Input: part model. Units: mm. Frame: model coordinates. A direction names the side the tool comes from. Give positions to 0.01 mm unless a question says otherwise; leave off trailing zeros. Loops run counter-clockwise (first coordinate to the right, second up) from the corner with the lowest first, then second, coordinate; pieces in that order, holes last. Notation, with made-up numbers: M 44.25,87 L 48.25,87 A23 cw 48.25,110 Z; hole C 58.5,25 d7. An arc over 180 degrees is marked long. One line per item, written item: value. Start each with the question number.
(1) Pin query (flat end, axial travel): P1, Ø0.9, axis at y = 2.5, z = 2, coming from the -X side; P2, Ø1.5, axis at x = 1.5, z = -1, coming from the +Y side; P3, Ø1.2, axis at x = -2.54, y = -4.43, coming from the -Z side. Return the tip coordinate at first contact, or that it passes through.
(2) Section C-C on x = -1. Output: boundary loops of the cut face in (y, z).
(3) Section B-B on y = -4.43. Output: boundary loops of the cut face in (x, z).
(4) Ray query, line 1 along Y through (x, z) = (0, 0.6); line 2 along X through (y, z) = (3.75, -1.05); line 3 along Z through (x, y) = (-2.25, -3). Return the intervals inside material, ascending. Write a range as from..to.
(5) Access query for faces 4 (the flat face through (0, 5.2, -1)), 5 (the flat face through (-3.3, 2, 2)), 6 (the flat face through (3.3, 2, -1)). Directions: +Z, -Z, +X, -X, +Y, -Y. A direction counts if a zero-diameter tool reaches every point of the face in a straight line with its end or side. Return the directions, or none.
(6) Section A-A on x = 0. Output: boundary loops of the cut face in (y, z), plus the area to 3 significant figures.
(7) Pull-direction query (X, two-part tool) for faces 1 (the flat face through (-3.3, 2, -1)), 2 (the cylindrical face through (-2.65, -3.93, 0.5)), 3 (the flat face through (0, 2, 2.82)); classes: released by +X, released by -X, zero draft, split by the parting line, or undercut.
(8) Section D-D on z = 2.4. Output: boundary loops of the cut face in (x, y).
Autodesk Inventor part; units mm, degrees
ref_plane "YZ Plane" through (0, 0, 0) normal (1, 0, 0) x (0, 1, 0)
ref_plane "XZ Plane" through (0, 0, 0) normal (0, 1, 0) x (-1, 0, 0)
ref_plane "XY Plane" through (0, 0, 0) normal (0, 0, 1) x (1, 0, 0)
sketch "スケッチ1" plane through (0, 0, 0) normal (0, 0, 1) x (1, 0, 0)
  line L0 (-3.8, -5.7) -> (3.8, -5.7)
  line L1 (3.8, -5.7) -> (3.8, 5.7)
  line L2 (3.8, 5.7) -> (-3.8, 5.7)
  line L3 (-3.8, 5.7) -> (-3.8, -5.7)
  line L4 (-3.8, -5.7) -> (3.8, 5.7) construction
  line L5 (3.8, -5.7) -> (-3.8, 5.7) construction
  circle A0 centre (0, -4.43) radius 0.51
  circle A1 centre (-2.54, -4.43) radius 0.51
  circle A2 centre (2.54, -4.43) radius 0.51
  point P0 (0, 0)
  point P1 (0, 0)
  dimension "d0" = 11.4
  dimension "d1" = 7.6
  dimension "d2" = 1.27
  dimension "d3" = 2.54
  dimension "d4" = 2.54
  dimension "d5" = 1.02
extrude "押し出し1" add sketch "スケッチ1" along normal blind 1.02
sketch "スケッチ2" plane through (0, 0, 1.02) normal (0, 0, 1) x (1, 0, 0)
  line L0 (-3.3, 5.2) -> (3.3, 5.2)
  line L1 (3.3, 5.2) -> (3.3, -0.8)
  line L2 (3.3, -0.8) -> (-3.3, -0.8)
  line L3 (-3.3, -0.8) -> (-3.3, 5.2)
  line L4 (-3.3, 5.2) -> (3.3, -0.8) construction
  line L5 (3.3, 5.2) -> (-3.3, -0.8) construction
  line L6 (3.8, 5.7) -> (-3.8, 5.7)
  line L7 (-3.8, 5.7) -> (-3.8, -5.7)
  line L8 (3.8, -5.7) -> (3.8, 5.7)
  point P0 (0, 0)
  point P1 (0, 2.2)
  dimension "d8" = 0.5
  dimension "d9" = 0.5
  dimension "d10" = 0.5
  dimension "d11" = 6
extrude "押し出し2" add sketch "スケッチ2" along normal blind 1.8
sketch "スケッチ3" plane through (0, 0, 0) normal (0, 0, -1) x (-1, 0, 0)
  line L0 (-3.3, 5.2) -> (3.3, 5.2)
  line L1 (3.3, 5.2) -> (3.3, -0.8)
  line L2 (3.3, -0.8) -> (-3.3, -0.8)
  line L3 (-3.3, -0.8) -> (-3.3, 5.2)
  point P0 (0, 0)
extrude "押し出し3" add sketch "スケッチ3" along normal blind 1.4
sketch "スケッチ4" plane through (0, 0, 1.02) normal (0, 0, 1) x (1, 0, 0)
  line L0 (-3.0991, -3.2712) -> (-1.8939, -3.2712) construction
  line L1 (-1.8939, -3.2712) -> (-1.8939, -3.8169) construction
  line L2 (-1.8939, -3.8169) -> (-3.0991, -3.8169) construction
  line L3 (-3.0991, -3.8169) -> (-3.0991, -3.2712) construction
  line L4 (-0.6641, -3.2466) -> (0.9346, -3.2466) construction
  line L5 (0.9346, -3.2466) -> (0.9346, -3.8169) construction
  line L6 (0.9346, -3.8169) -> (-0.6641, -3.8169) construction
  line L7 (-0.6641, -3.8169) -> (-0.6641, -3.2466) construction
  line L8 (1.7955, -3.2958) -> (3.5455, -3.2958) construction
  line L9 (3.5455, -3.2958) -> (3.5455, -3.8169) construction
  line L10 (3.5455, -3.8169) -> (1.7955, -3.8169) construction
  line L11 (1.7955, -3.8169) -> (1.7955, -3.2958) construction
  point P0 (0, 0)
properties part number "S7V7F5"
Output values:
1. P1: stops at x = -3.3
1. P2: stops at y = 5.2
1. P3: stops at z = 0
2. outline: M -5.7,0 L -0.8,0 L -0.8,-1.4 L 5.2,-1.4 L 5.2,0 L 5.7,0 L 5.7,1.02 L 5.2,1.02 L 5.2,2.82 L -0.8,2.82 L -0.8,1.02 L -5.7,1.02 Z
3. outline: M -3.8,0 L -3.05,0 L -3.05,1.02 L -3.8,1.02 Z; M -2.03,0 L -0.51,0 L -0.51,1.02 L -2.03,1.02 Z; M 0.51,0 L 2.03,0 L 2.03,1.02 L 0.51,1.02 Z; M 3.05,0 L 3.8,0 L 3.8,1.02 L 3.05,1.02 Z
4. line 1: y = -5.7..-4.94, -3.92..5.7
4. line 2: x = -3.3..3.3
4. line 3: z = 0..1.02
5. face 4: -Z, +X, -X, +Y
5. face 5: +Z, -X, +Y, -Y
5. face 6: -Z, +X, +Y, -Y
6. outline: M -5.7,0 L -4.94,0 L -4.94,1.02 L -5.7,1.02 Z; M -3.92,0 L -0.8,0 L -0.8,-1.4 L 5.2,-1.4 L 5.2,0 L 5.7,0 L 5.7,1.02 L 5.2,1.02 L 5.2,2.82 L -0.8,2.82 L -0.8,1.02 L -3.92,1.02 Z
6. area: 29.8 mm²
7. face 1: released by -X
7. face 2: undercut
7. face 3: zero draft
8. outline: M -3.3,-0.8 L 3.3,-0.8 L 3.3,5.2 L -3.3,5.2 Z
